```python
from build123d import *

# Parameters (mm, degrees)
SKETCH1_W           = 63.5
SKETCH1_H           = 25.4
BOSS_EXTRUDE1_DEPTH = 38.1
SKETCH2_R           = 3.175
CUT_EXTRUDE1_DEPTH  = 12.7
SKETCH2_3_R         = 8.763
CUT_EXTRUDE2_DEPTH  = 4.826
CUT_EXTRUDE3_START  = -20.574
SKETCH3_R           = 6.35
CUT_EXTRUDE3_DEPTH  = 20.574
SKETCH4_R           = 10.795
CUT_EXTRUDE4_DEPTH  = 19.05
SKETCH5_R           = 1.5875
CUT_EXTRUDE5_DEPTH  = 50.8
SKETCH6_W           = 63.5
SKETCH6_H           = 1.27
CUT_EXTRUDE6_DEPTH  = 38.1
SKETCH7_W           = 63.5
SKETCH7_H           = 24.13
BOSS_EXTRUDE2_DEPTH = 1.524


with BuildPart() as part:
    # Sketch1 → Boss-Extrude1 (new body)
    with BuildSketch(Plane.XY):
        Rectangle(SKETCH1_W, SKETCH1_H)
    extrude(amount=BOSS_EXTRUDE1_DEPTH)

    # Sketch2 → Cut-Extrude1 (cut)
    with BuildSketch(Plane.XZ.offset(12.7)):
        with Locations(Location((-24.765, 15.24, 0), (0, 0, 270))):
            Circle(SKETCH2_R)
        with Locations(Location((24.765, 15.24, 0), (0, 0, 270))):
            Circle(SKETCH2_R)
    extrude(amount=-CUT_EXTRUDE1_DEPTH, mode=Mode.SUBTRACT)

    # Sketch2<3> → Cut-Extrude2 (cut)
    with BuildSketch(Plane.XZ.offset(12.7)):
        with Locations(Location((0, 15.24, 0), (0, 0, 270))):
            Circle(SKETCH2_3_R)
    extrude(amount=-CUT_EXTRUDE2_DEPTH, mode=Mode.SUBTRACT)

    # Sketch3 → Cut-Extrude3 (cut)
    with BuildSketch(Plane.XZ.offset(7.874).offset(CUT_EXTRUDE3_START)):
        with Locations(Location((0, 15.24, 0), (0, 0, 270))):
            Circle(SKETCH3_R)
    extrude(amount=CUT_EXTRUDE3_DEPTH, mode=Mode.SUBTRACT)

    # Sketch4 → Cut-Extrude4 (cut)
    with BuildSketch(Plane(origin=(0, 12.7, 0), x_dir=(1, 0, 0), z_dir=(0, 1, 0))):
        with Locations(Location((0, -15.24, 0), (0, 0, 270))):
            Circle(SKETCH4_R)
    extrude(amount=-CUT_EXTRUDE4_DEPTH, mode=Mode.SUBTRACT)

    # Sketch5 → Cut-Extrude5 (cut)
    with BuildSketch(Plane(origin=(0, 12.7, 0), x_dir=(1, 0, 0), z_dir=(0, 1, 0))):
        with Locations(Location((-26.67, -34.925, 0), (0, 0, 270))):
            Circle(SKETCH5_R)
        with Locations(Location((0, -34.925, 0), (0, 0, 270))):
            Circle(SKETCH5_R)
        with Locations(Location((26.67, -34.925, 0), (0, 0, 270))):
            Circle(SKETCH5_R)
    extrude(amount=-CUT_EXTRUDE5_DEPTH, mode=Mode.SUBTRACT)

    # Sketch6 → Cut-Extrude6 (cut)
    with BuildSketch(Plane.XY.offset(38.1)):
        with Locations((0, -12.065)):
            Rectangle(SKETCH6_W, SKETCH6_H)
    extrude(amount=-CUT_EXTRUDE6_DEPTH, mode=Mode.SUBTRACT)

    # Sketch7 → Boss-Extrude2 (add)
    with BuildSketch(Plane.XY.offset(38.1)):
        with Locations((0, 0.635)):
            Rectangle(SKETCH7_W, SKETCH7_H)
    extrude(amount=BOSS_EXTRUDE2_DEPTH)


solid = part.part
```
CAD build for the part. Positions are in the model's coordinates, mm. A direction names the side the tool comes from. Coordinates: 2 decimals unless noted, no trailing zeros. Write each loop counter-clockwise with the first axis right and the second up, starting at its lowest first coordinate (ties: lowest second). Pieces come first, ordered by that corner, then holes. Notation, with made-up numbers: (60.25, -22) -> (85.25, -22) arc R29 cw to (85.25, 6) -> close; hole circle Ø4 at (-26.5, 21.25). An arc over 180 degrees is marked (long way). Use CSV: the item, a comma, the result in double quotes. Start each with the question number.
Item 1: Band-saw the part on A-A, the plane x = 26.67. Write the cut outline in (y, z), plus the area to 3 significant figures.
Item 2: Band-saw the part on B-B, the plane z = 15.24. Write the cut outline in (x, y) (3 decimals), plus the area to 3 significant figures.
Item 3: Band-saw the part on C-C, the plane y = 8. Give the number of separate pieces and of enclosed holes in the cut face, plus the area to 3 significant figures.
Item 4: Wall check: probe 1 along X at (y, z) = (-10.45, 15.24); probe 2 along X at (y, z) = (-1.25, 15.5); probe 3 along X at (y, z) = (-5.5, 7.5). Give the ranges that are in metal, low to high.
Item 5: Drop flat-ended pins along their axis: P1, Ø3, axis at x = -26, z = 15.5, coming from the -Y side; P2, Ø14.5, axis at x = 0, z = 15.24, coming from the +Y side; P3, Ø5.5, axis at x = -4.5, z = 12, coming from the -Y side. Give the stop position or say it passes through.
Item 6: Two-plate mould, pull along Z, no slides. Class faces 1 (the flat face through (0, 1, 39.624)), 2 (the cylindrical face through (28.244, 0.804, 34.718)), 3 (the flat face through (-8, -11.43, 24)), 4 (the cylindrical face through (3.243, 3.308, 25.537)): +Z half, -Z half, draft (parallel to the pull), parting line (faces both ways), or undercut.
Item 7: Tool access for faces 5 (the flat face through (-5, -6.35, 20)), 6 (the flat face through (0, 1, 0)), 7 (the cylindrical face through (2.63, -9.68, 6.88)): list every direction of +Z, -Z, +X, -X, +Y, -Y with a clear straight run to the whole face (end or side of a thin tool).
Response values:
1,outline,"(-11.43, 0) -> (12.7, 0) -> (12.7, 33.34) -> (-11.43, 33.34) -> (-11.43, 17.78) -> (0, 17.78) -> (0, 12.7) -> (-11.43, 12.7) -> close; (-11.43, 36.51) -> (12.7, 36.51) -> (12.7, 39.62) -> (-11.43, 39.62) -> close"
1,area,"821 mm2"
2,outline,"(-31.75, -11.43) -> (-27.94, -11.43) -> (-27.94, 0) -> (-21.59, 0) -> (-21.59, -11.43) -> (-8.763, -11.43) -> (-8.763, -7.874) -> (-6.35, -7.874) -> (-6.35, -6.35) -> (-10.795, -6.35) -> (-10.795, 12.7) -> (-31.75, 12.7) -> close; (6.35, -7.874) -> (8.763, -7.874) -> (8.763, -11.43) -> (21.59, -11.43) -> (21.59, 0) -> (27.94, 0) -> (27.94, -11.43) -> (31.75, -11.43) -> (31.75, 12.7) -> (10.795, 12.7) -> (10.795, -6.35) -> (6.35, -6.35) -> close"
2,area,"894 mm2"
3,separate pieces,"1"
3,enclosed holes,"4"
3,area,"2,130 mm2"
4,probe 1,"x = -31.75 to -27.94, -21.59 to -8.76, 8.76 to 21.59, 27.94 to 31.75"
4,probe 2,"x = -31.75 to -27.93, -21.6 to -10.79, 10.79 to 21.6, 27.93 to 31.75"
4,probe 3,"x = -31.75 to -7.52, 7.52 to 31.75"
5,P1,"stops at y = 0"
5,P2,"stops at y = -6.35"
5,P3,"stops at y = -7.87"
6,face 1,"+Z half"
6,face 2,"undercut"
6,face 3,"draft"
6,face 4,"undercut"
7,face 5,"+Y"
7,face 6,"-Z, +X, -X, +Y, -Y"
7,face 7,"-Y"
